Read the model definition and answer for the solid it produces. Units are mm, in the model's axes. Coordinates: 2 decimals unless noted, no trailing zeros. Write each loop counter-clockwise with the first axis right and the second up, starting at its lowest first coordinate (ties: lowest second). Pieces come first, ordered by that corner, then holes. Notation, with made-up numbers: (-26, 61) -> (-10, 61) arc R24 cw to (-10, 72) -> close; hole circle Ø4 at (21, -21). An arc over 180 degrees is marked (long way). Answer as a JSON object with one key per item and string values. Group by question number.
(1) Find section A-A (z = 40). Give the vertices of the cut face in (x, y), then the cut area to 3 significant figures.
(2) For a pull along Z with two mould halves and no side action, classify faces 1 (the face through (1, 0, 31)), 2 (the face through (-7.493, -0.33, 0.159)), 3 (the face through (0, 0, -11.925)), 4 (the face through (3.251, -1.024, 11.983)) as +Z half, -Z half, draft (parallel to the pull), parting line (faces both ways), or undercut.
(3) Straight lines are drawn through the part: L1, parallel to Z at x = 5.5, y = -3.5 (3 decimals); L2, parallel to Z at x = -4.75, y = 1.5 (3 decimals); L3, parallel to X at y = -3.25, z = 10. For each, find the intervals that lie inside material, in ascending order.
(4) Find section B-B (z = -2.5). Give the vertices of the cut face in (x, y), then the cut area to 3 significant figures.
(5) Flat-ended cylindrical pins translate along their axes: P1, Ø6, axis at y = -3.5, z = 34, coming from the -X side; P2, Ø8, axis at x = -3, z = 25.5, coming from the +Y side; P3, Ø1.5, axis at x = -1.5, z = -3, coming from the -Y side. Find the tip coordinate at first contact, or state that the pin passes through.
from build123d import *

# Parameters (mm, degrees)
SKETCH2_R           = 1
BOSS_EXTRUDE1_DEPTH = 30
FILLET1_R           = 5


with BuildPart() as part:
    # Sketch1 → Revolve1 (revolve)
    with BuildSketch(Plane(origin=(0, 0, 0), x_dir=(1, 0, 0), z_dir=(0, 1, 0))):
        Polygon((0, 0), (0, 11.925), (2.5, 11.925), (2.5, 5.925), (7.5, 5.925), (7.5, -6.075), (1, -15.460714286), (0, -15.460714286), align=None)
    revolve(axis=Axis((0, 0, 0), (0, 0, -1)))

    # Sketch2 → Boss-Extrude1 (add)
    with BuildSketch(Plane.XY.offset(15.460714286)):
        Circle(SKETCH2_R)
    extrude(amount=BOSS_EXTRUDE1_DEPTH)

    # Fillet1
    fillet1_edges = [part.edges().sort_by_distance(p)[0] for p in [
        (-1, 0, 15.460714286),
    ]]
    fillet(fillet1_edges, radius=FILLET1_R)

    # Sketch4 → Revolve8 (revolve)
    with BuildSketch(Plane(origin=(0, 0, 46.460714286), x_dir=(-1, 0, 0), z_dir=(0, 0, -1))):
        with BuildLine():
            Line((-1.5, 0), (1.5, 0))
            ThreePointArc((1.5, 0), (0, -1.5), (-1.5, 0))
        make_face()
    revolve(axis=Axis((-1.5, 0, 46.460714286), (1, 0, 0)))


solid = part.part
Results below:
{
 "1": {"outline": "circle Ø2 at (0, 0)", "area": "3.14 mm2"},
 "2": {"face 1": "undercut", "face 2": "draft", "face 3": "-Z half", "face 4": "+Z half"},
 "3": {"L1": "z = -5.925 to 7.491", "L2": "z = -5.925 to 9.712", "L3": "x = -3.51 to 3.51"},
 "4": {"outline": "circle Ø15 at (0, 0)", "area": "177 mm2"},
 "5": {"P1": "stops at x = -0.87", "P2": "stops at y = 1", "P3": "stops at y = -7.46"}
}
